Verification items for the finished model (mm, model axes). A direction names the side the tool comes from. Give positions to 0.01 mm unless a question says otherwise; leave off trailing zeros. Write each loop counter-clockwise with the first axis right and the second up, starting at its lowest first coordinate (ties: lowest second). Pieces come first, ordered by that corner, then holes. Notation, with made-up numbers: (35.25, 3.25) -> (52.25, 3.25) arc R24 ccw to (52.25, 36.25) -> close; hole circle Ø5 at (22, 50.25). An arc over 180 degrees is marked (long way). Write item = value, one per line.
from build123d import *

# Parameters (mm, degrees)
SKETCH1_R           = 7.575
BOSS_EXTRUDE1_DEPTH = 5.2
CUT_EXTRUDE1_DEPTH  = 3.6
BOSS_EXTRUDE2_DEPTH = 16.4
FILLET1_R           = 1
BOSS_EXTRUDE3_DEPTH = 4.85
SKETCH6_R           = 1.875
BOSS_EXTRUDE4_DEPTH = 2.55
CUT_EXTRUDE2_DEPTH  = 4


with BuildPart() as part:
    # Sketch1 → Boss-Extrude1 (new body)
    with BuildSketch(Plane(origin=(0, 0, 0), x_dir=(1, 0, 0), z_dir=(0, 1, 0))):
        Circle(SKETCH1_R)
    extrude(amount=BOSS_EXTRUDE1_DEPTH)

    # Sketch2 → Cut-Extrude1 (cut)
    with BuildSketch(Plane.XZ):
        with BuildLine():
            Line((-4.359330502, -1.388114754), (0, -4.575))
            ThreePointArc((0, -4.575), (2.7, 3.693321676), (-4.359330502, -1.388114754))
        make_face()
    extrude(amount=-CUT_EXTRUDE1_DEPTH, mode=Mode.SUBTRACT)

    # Sketch4 → Boss-Extrude2 (add)
    with BuildSketch(Plane(origin=(0, 5.2, 0), x_dir=(1, 0, 0), z_dir=(0, 1, 0))):
        Polygon((6.611448404, 0), (0, 6.611448404), (-6.611448404, 0), (0, -6.611448404), align=None)
        Polygon((4.242640687, 0), (0, 4.242640687), (-4.242640687, 0), (0, -4.242640687), align=None, mode=Mode.SUBTRACT)
    extrude(amount=BOSS_EXTRUDE2_DEPTH)

    # Fillet1
    fillet1_edges = [part.edges().sort_by_distance(p)[0] for p in [
        (3.305724202, 21.6, 3.305724202),
        (3.305724202, 21.6, -3.305724202),
        (-3.305724202, 21.6, -3.305724202),
        (-3.305724202, 21.6, 3.305724202),
        (0, 13.4, 6.611448404),
        (6.611448404, 13.4, 0),
        (0, 13.4, -6.611448404),
        (-6.611448404, 13.4, 0),
    ]]
    fillet(fillet1_edges, radius=FILLET1_R)

    # Sketch5 → Boss-Extrude3 (add)
    with BuildSketch(Plane(origin=(0, 5.2, 0), x_dir=(1, 0, 0), z_dir=(0, 1, 0))):
        Polygon((0, -4.242640687), (4.242640687, 0), (0, 4.242640687), (-4.242640687, 0), align=None)
    extrude(amount=BOSS_EXTRUDE3_DEPTH)

    # Sketch6 → Boss-Extrude4 (add)
    with BuildSketch(Plane(origin=(0, 10.05, 0), x_dir=(1, 0, 0), z_dir=(0, 1, 0))):
        Circle(SKETCH6_R)
    extrude(amount=BOSS_EXTRUDE4_DEPTH)

    # Sketch3 → Cut-Extrude2 (cut)
    with BuildSketch(Plane.XZ.offset(-3.6)):
        with BuildLine():
            Line((-1.9, 2.157689737), (1.9, 2.157689737))
            ThreePointArc((1.9, 2.157689737), (0, -2.875), (-1.9, 2.157689737))
        make_face()
    extrude(amount=-CUT_EXTRUDE2_DEPTH, mode=Mode.SUBTRACT)


solid = part.part
Item 1: Material ranges on line 1 (X direction, y = 5.15, z = 0) (3 decimals); line 2 (X direction, y = 2.5, z = 0) (3 decimals); line 3 (Y direction, x = -1.25, z = -1.25), recorded low to high.
Response values:
line_1 = -7.575 to -2.875, 2.875 to 7.575
line_2 = -7.575 to -4.575, 4.575 to 7.575
line_3 = 7.6 to 12.6
Item 2: Set-up check for faces 1 (the cylindrical face through (-6.197, 13.008, -0.011)), 2 (the flat face through (-2.21, 1.77, -2.96)), 3 (the cylindrical face through (-1.873, 11.307, -0.082)): record each of +Z, -Z, +X, -X, +Y, -Y from which the full face is reachable in a straight line by a thin tool's end or side.
Response values:
face_1 = -X, +Y
face_2 = -Y
face_3 = +Y
Item 3: Sectioned sample at B-B on y = 7. Record the cut outline in (x, z) (3 decimals).
Response values:
outline = (-5.904, -0.707) -> (-0.707, -5.904) arc R1 ccw to (0.707, -5.904) -> (5.904, -0.707) arc R1 ccw to (5.904, 0.707) -> (0.707, 5.904) arc R1 ccw to (-0.707, 5.904) -> (-5.904, 0.707) arc R1 ccw to start; hole (-1.9, 2.158) arc R2.875 ccw (long way) to (1.9, 2.158) -> close
Item 4: Sectioned sample at A-A on y = 12. Record the cut outline in (x, z) (3 decimals).
Response values:
outline = (-5.904, -0.707) -> (-0.707, -5.904) arc R1 ccw to (0.707, -5.904) -> (5.904, -0.707) arc R1 ccw to (5.904, 0.707) -> (0.707, 5.904) arc R1 ccw to (-0.707, 5.904) -> (-5.904, 0.707) arc R1 ccw to start; circle Ø3.75 at (0, 0); hole (-4.243, 0) -> (0, -4.243) -> (4.243, 0) -> (0, 4.243) -> close
Item 5: Mould release check, pull along X, two halves, no side actions. Record for faces 4 (the flat face through (0, 12.6, 0)), 5 (the flat face through (-3.34, 12.79, 3.27)), 6 (the cylindrical face through (3.14, 21.3, 3.07)): +X half, -X half, draft (parallel to the pull), parting line (faces both ways), or undercut.
Response values:
face_4 = undercut
face_5 = -X half
face_6 = +X half
Item 6: Go/stop test with flat-tipped pins: P1, Ø3, axis at x = -1, y = 12, coming from the +Z side; P2, Ø1.5, axis at x = 1.5, z = 1, coming from the +Y side; P3, Ø4, axis at x = 4.5, y = 15.5, coming from the +Z side. Record where each tip stops, or that it passes through.
Response values:
P1 = 6.2
P2 = 12.6
P3 = 4.11
